Check sheet for the drawn part. Datum: minimum x, y, z corner. Units: mm. Round coordinates to 2 decimals unless told otherwise and drop trailing zeros. Write each loop counter-clockwise with the first axis right and the second up, starting at its lowest first coordinate (ties: lowest second). Pieces come first, ordered by that corner, then holes. Notation, with made-up numbers: (57, 73) -> (111, 73) arc R12 cw to (111, 89) -> close; hole circle Ø3 at (17, 76). An arc over 180 degrees is marked (long way). One line per item, written item: value.
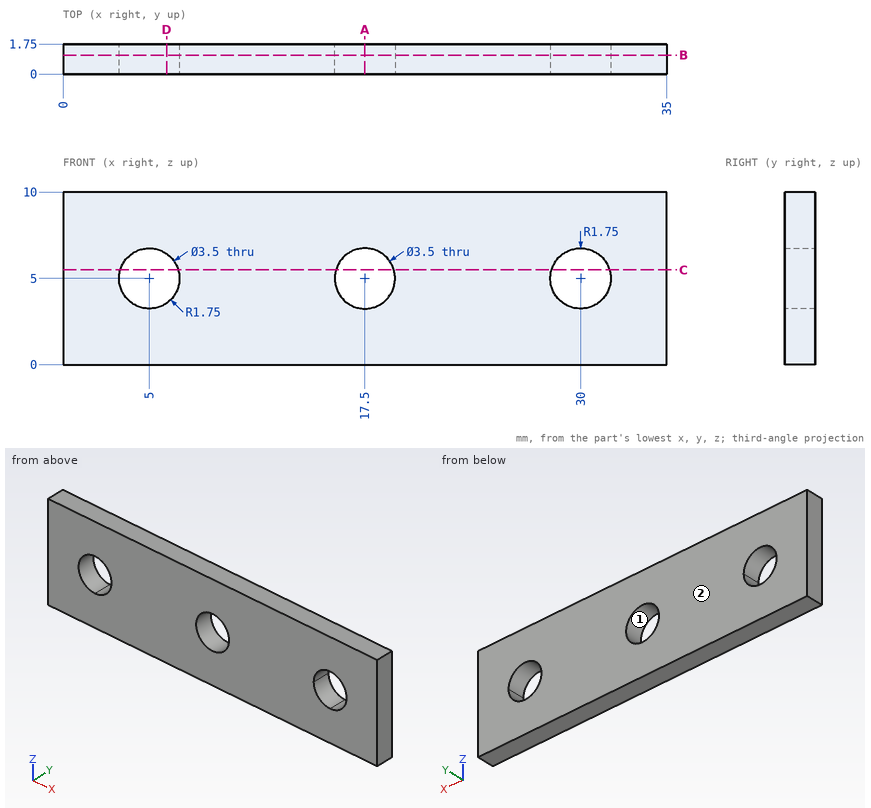
Item 1: Sectioned sample at C-C on z = 5.5. Enter the section's corners in (x, y).
Answer:
outline: (0, 0) -> (3.32, 0) -> (3.32, 1.75) -> (0, 1.75) -> close; (6.68, 0) -> (15.82, 0) -> (15.82, 1.75) -> (6.68, 1.75) -> close; (19.18, 0) -> (28.32, 0) -> (28.32, 1.75) -> (19.18, 1.75) -> close; (31.68, 0) -> (35, 0) -> (35, 1.75) -> (31.68, 1.75) -> close
Item 2: Sectioned sample at D-D on x = 6. Enter the section's corners in (y, z).
Answer:
outline: (0, 0) -> (1.75, 0) -> (1.75, 3.56) -> (0, 3.56) -> close; (0, 6.44) -> (1.75, 6.44) -> (1.75, 10) -> (0, 10) -> close
Item 3: Sectioned sample at A-A on x = 17.5. Enter the section's corners in (y, z), and give its area (3 significant figures).
Answer:
outline: (0, 0) -> (1.75, 0) -> (1.75, 3.25) -> (0, 3.25) -> close; (0, 6.75) -> (1.75, 6.75) -> (1.75, 10) -> (0, 10) -> close
area: 11.4 mm^2
Item 4: Mould release check, pull along X, two halves, no side actions. Record for the marked faces 1 and 2: pulls with the +X half, pulls with the -X half, needs draft (parallel to the pull), parting line crosses it, or undercut.
Answer:
face 1: undercut
face 2: needs draft
Item 5: Sectioned sample at B-B on y = 1.1. Enter the section's corners in (x, z), and give its area (3 significant figures).
Answer:
outline: (0, 0) -> (35, 0) -> (35, 10) -> (0, 10) -> close; hole circle Ø3.5 at (5, 5); hole circle Ø3.5 at (17.5, 5); hole circle Ø3.5 at (30, 5)
area: 321 mm^2
Item 6: Thickness scan on line 1 (Z direction, x = 5, y = 0.6); line 2 (X direction, y = 0.85, z = 5.5); line 3 (X direction, y = 0.85, z = 6.25). Record the ranges inside material, lowest first.
Answer:
line 1: z = 0 to 3.25, 6.75 to 10
line 2: x = 0 to 3.32, 6.68 to 15.82, 19.18 to 28.32, 31.68 to 35
line 3: x = 0 to 3.78, 6.22 to 16.28, 18.72 to 28.78, 31.22 to 35
